Autodesk Inventor part; units mm, degrees
ref_plane "YZ Plane" through (0, 0, 0) normal (1, 0, 0) x (0, 1, 0)
ref_plane "XZ Plane" through (0, 0, 0) normal (0, 1, 0) x (-1, 0, 0)
ref_plane "XY Plane" through (0, 0, 0) normal (0, 0, 1) x (1, 0, 0)
sketch "Sketch1" plane through (0, 0, 0) normal (0, 1, 0) x (-1, 0, 0)
  line L0 (-16, 35) -> (21, 35)
  line L1 (21, 35) -> (21, -35)
  line L2 (21, -35) -> (-16, -35)
  line L3 (-21, -30) -> (-21, 30)
  line L4 (-21, 35) -> (21, -35) construction
  line L5 (21, 35) -> (-21, -35) construction
  line L6 (-36, -15) -> (-6, -15)
  line L7 (-6, -15) -> (-6, 15)
  line L8 (-6, 15) -> (-36, 15)
  line L9 (-36, 15) -> (-36, -15)
  line L10 (-36, -15) -> (-6, 15) construction
  line L11 (-6, -15) -> (-36, 15) construction
  line L12 (-16, -35) -> (-21, -30)
  line L13 (-21, 30) -> (-16, 35)
  point P0 (0, 0)
  point P1 (-21, 0)
  point P2 (-21, -15)
  point P3 (-21, 15)
  dimension "d0" = 42
  dimension "d1" = 70
  dimension "d10" = 30
  dimension "d11" = 30
  dimension "d12" = 5
  dimension "d13" = 5
  dimension "d14" = 5
  dimension "d15" = 5
extrude "Extrusion1" add sketch "Sketch1" along normal blind 2
fillet "Fillet1" radius 3 10 edges at (36, 1, -15) (36, 1, 15) (21, 1, -30) (16, 1, -35) (21, 1, 30) (16, 1, 35) (-21, 1, 35) (-21, 1, -35) (21, 1, -15) (21, 1, 15)
equation "\"d13\" = d12"
equation "\"d14\" = d12"
equation "\"d15\" = d14"
properties part number "Second Layer Board"
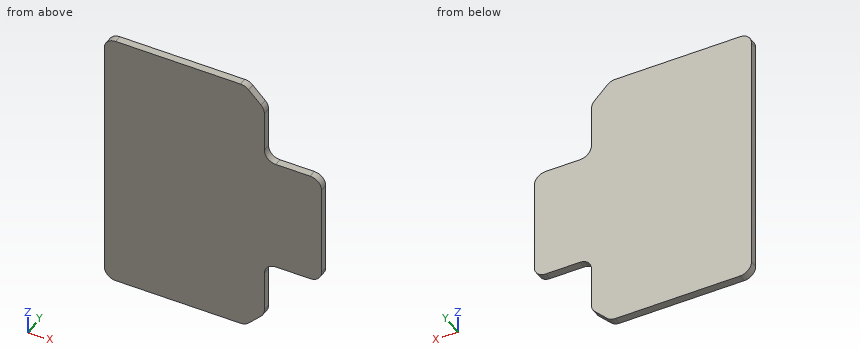
Check sheet for the modelled part. Datum: model origin and axes. Units: mm. Round coordinates to 2 decimals unless told otherwise and drop trailing zeros. Loops run counter-clockwise (first coordinate to the right, second up) from the corner with the lowest first, then second, coordinate; pieces in that order, holes last. Notation, with made-up numbers: (81, 29) - (129, 29) arc R17 ccw to (129, 37) - close; hole circle Ø6 at (33.25, 13). An arc over 180 degrees is marked (long way). Answer as a JSON object with one key per item and string values. Group by question number.
Q1. Scan lines: line 1 along Z through (x, y) = (30.5, 1); line 2 along X through (y, z) = (1.95, 18.5); line 3 along Z through (x, y) = (23, 1.25). Record each from-to range of solid material in increasing order. Write a range as [from, to].
Q2. Gauge pin test, flat ends, axial feed: P1, Ø0.6, axis at y = 1, z = 22, coming from the +X side; P2, Ø1, axis at x = 27.5, y = 0.5, coming from the +Z side; P3, Ø1, axis at x = 27.5, y = 0.5, coming from the -Z side. Record the tip position at first contact, or that the pin passes through.
Q3. Sectioned sample at B-B, the plane z = 26. Enter the section's corners in (x, y).
Q4. Sectioned sample at A-A, the plane y = 1.7. Enter the section's corners in (x, z), plus the area to 3 significant figures.
Solution:
{
 "1": {"line 1": "z = [-15, 15]", "line 2": "x = [-21, 21]", "line 3": "z = [-15.17, 15.17]"},
 "2": {"P1": "stops at x = 21", "P2": "stops at z = 15", "P3": "stops at z = -15"},
 "3": {"outline": "(-21, 0) - (21, 0) - (21, 2) - (-21, 2) - close"},
 "4": {"outline": "(-21, -32) arc R3 ccw to (-18, -35) - (14.76, -35) arc R3 ccw to (16.88, -34.12) - (20.12, -30.88) arc R3 ccw to (21, -28.76) - (21, -18) arc R3 cw to (24, -15) - (33, -15) arc R3 ccw to (36, -12) - (36, 12) arc R3 ccw to (33, 15) - (24, 15) arc R3 cw to (21, 18) - (21, 28.76) arc R3 ccw to (20.12, 30.88) - (16.88, 34.12) arc R3 ccw to (14.76, 35) - (-18, 35) arc R3 ccw to (-21, 32) - close", "area": "3,360 mm²"}
}
